For this review, take the finished solid that the model builds, in its own axes (mm). Face numbers are marked on the shaded views. A direction names the side the tool comes from. Coordinates: 2 decimals unless noted, no trailing zeros. Loops run counter-clockwise (first coordinate to the right, second up) from the corner with the lowest first, then second, coordinate; pieces in that order, holes last. Notation, with made-up numbers: (-3, 60.25) - (24, 60.25) arc R18 ccw to (24, 87.25) - close; hole circle Ø11 at (-33, 69.5). An arc over 180 degrees is marked (long way). Answer as a JSON object with one key per item and string values. Group by question number.
Item 1: Mouldability with a two-part tool opening along X and no side actions: class the marked faces 1, 2 and 3 as released by +X, released by -X, zero draft, split by the parting line, or undercut.
Item 2: Clearance check with flat-ended pins moving along their axes: pin 1 (2.5 mm diameter, centred on x = 8.5, y = -19, fed in from -Z) (3 decimals); pin 2 (12 mm diameter, centred on x = 26, z = 9, fed in from +Y); pin 3 (5 mm diameter, centred on x = 19, z = 14.5, fed in from -Y). State where each tip first meets the part, or that it passes through.
Item 3: We need section D-D (z = 13). Give the boundary of the cut face in (x, y), then the cut area to 3 significant figures.
Item 4: We need section B-B (y = -26). Give the boundary of the cut face in (x, z) (3 decimals).
Item 5: To check wall thickness, follow line 1 (Y direction, x = 13.5, z = 18); line 2 (X direction, y = -28, z = 26); line 3 (X direction, y = -31, z = 26.5). State the ranges of each line that lie inside material, in increasing order.
Item 6: We need section C-C (x = 8). Give the boundary of the cut face in (y, z) (3 decimals), then the cut area to 3 significant figures.
Item 7: We need section A-A (z = 8.5). Give the boundary of the cut face in (x, y), then the cut area to 3 significant figures.
Item 8: Tool access review of the marked faces 4, 5 and 6: name each direction out of +Z, -Z, +X, -X, +Y, -Y from which nothing blocks a thin tool from reaching the whole face with its end or side.
from build123d import *

# Parameters (mm, degrees)
F0_W     = 38.1
F0_H     = 38.1
F1_DEPTH = 38.1
F6_DEPTH = 38.1
F8_DEPTH = 38.1


with BuildPart() as f1:
    # F0 (on Front) → F1 (new body)
    with BuildSketch(Plane.XZ):
        with Locations((19.05, 19.05)):
            Rectangle(F0_W, F0_H)
    extrude(amount=F1_DEPTH)

    # F5 (on offset) → F6 (cut)
    with BuildSketch(Plane.XZ.offset(38.1)):
        Polygon((0, 38.1), (0, 0), (6.35, 0), align=None)
        Polygon((31.75, 38.1), (6.35, 38.1), (11.43, 15.77707), (16.51, 28.575), (21.59, 28.575), (26.67, 15.875), align=None)
        Polygon((38.1, 0), (38.1, 38.1), (31.75, 0), align=None)
        Polygon((19.05, 15.875), (12.7, 0), (25.4, 0), align=None)
    extrude(amount=-F6_DEPTH, mode=Mode.SUBTRACT)

    # F7 (on offset) → F8 (cut)
    with BuildSketch(Plane.YZ.offset(38.1)):
        Polygon((-38.1, 38.1), (-38.1, 0), (-31.784967, 38.1), align=None)
        Polygon((-26.67, 22.225), (-31.75, 0), (-6.35, 0), (-11.43, 22.225), (-16.51, 9.525), (-21.59, 9.525), align=None)
        Polygon((-12.780962, 38.1), (-25.4, 38.1), (-19.05, 22.225), align=None)
        Polygon((-6.315033, 38.1), (0, 0), (0, 38.1), align=None)
    extrude(amount=-F8_DEPTH, mode=Mode.SUBTRACT)


solid = f1.part
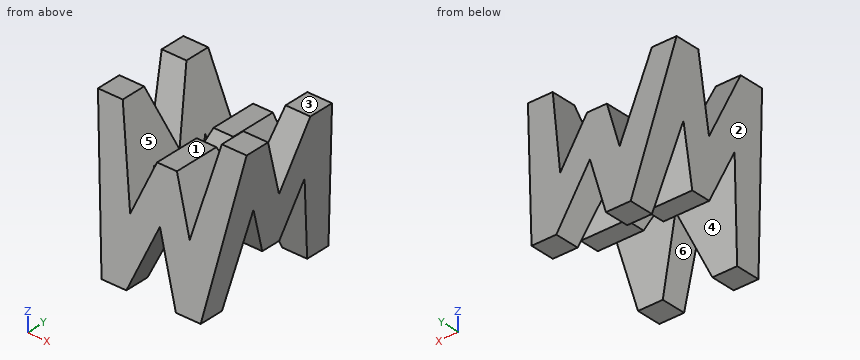
Check sheet entries:
{
 "1": {"face 1": "undercut", "face 2": "released by -X", "face 3": "zero draft"},
 "2": {"pin 1": "stops at z = 9.525", "pin 2": "stops at y = -0.5", "pin 3": "stops at y = -36.05"},
 "3": {"outline": "(4.18, -35.95) - (17.9, -35.95) - (17.9, -28.78) - (4.18, -28.78) - close; (4.18, -22.98) - (17.9, -22.98) - (17.9, -15.12) - (4.18, -15.12) - close; (4.18, -9.32) - (17.9, -9.32) - (17.9, -2.15) - (4.18, -2.15) - close; (20.2, -35.95) - (33.92, -35.95) - (33.92, -28.78) - (20.2, -28.78) - close; (20.2, -22.98) - (33.92, -22.98) - (33.92, -15.12) - (20.2, -15.12) - close; (20.2, -9.32) - (33.92, -9.32) - (33.92, -2.15) - (20.2, -2.15) - close", "area": "609 mm2"},
 "4": {"outline": "(0, 38.1) - (2.925, 20.55) - (10.344, 20.55) - (6.35, 38.1) - close; (13.325, 20.55) - (24.8, 20.55) - (21.59, 28.575) - (16.51, 28.575) - close; (27.739, 20.55) - (35.175, 20.55) - (38.1, 38.1) - (31.75, 38.1) - close"},
 "5": {"line 1": "y = -35.12 to -27.64, -24.98 to -13.12, -10.46 to -2.98", "line 2": "x = 2.02 to 9.1, 15.49 to 22.62, 28.98 to 36.08", "line 3": "x = 1.93 to 8.99, 15.69 to 22.42, 29.1 to 36.17"},
 "6": {"outline": "(-38.1, 0) - (-31.75, 0) - (-26.67, 22.225) - (-21.59, 9.525) - (-16.51, 9.525) - (-11.43, 22.225) - (-6.35, 0) - (0, 0) - (-5.113, 30.849) - (-15.644, 30.849) - (-19.05, 22.225) - (-22.5, 30.849) - (-32.987, 30.849) - close", "area": "665 mm2"},
 "7": {"outline": "(4.93, -36.69) - (16.1, -36.69) - (16.1, -29.81) - (4.93, -29.81) - close; (4.93, -8.29) - (16.1, -8.29) - (16.1, -1.41) - (4.93, -1.41) - close; (22, -36.69) - (33.17, -36.69) - (33.17, -29.81) - (22, -29.81) - close; (22, -8.29) - (33.17, -8.29) - (33.17, -1.41) - (22, -1.41) - close", "area": "307 mm2"},
 "8": {"face 4": "-Z, +X, -X", "face 5": "+Z, +Y, -Y", "face 6": "-Z, +Y, -Y"}
}
